Build history of the part. All positions in model axes, mm. Coordinates: 2 decimals unless noted, no trailing zeros. Loops run counter-clockwise (first coordinate to the right, second up) from the corner with the lowest first, then second, coordinate; pieces in that order, holes last.
(1) Slice it at D-D (z = 1.4). Give the cut face in (x, y), and give its area (3 significant figures).
(2) Slice it at C-C (y = -0.25). Give the cut face in (x, z), and give its area (3 significant figures).
(3) Wall check: L1, parallel to X at y = -0.1, z = 0; L2, parallel to Z at x = 14, y = 0.2; L3, parallel to X at y = 0.4, z = -1.05. Give the ranges that are in metal, low to high.
(4) Slice it at A-A (z = 0). Give the cut face in (x, y), and give its area (3 significant figures).
(5) Slice it at B-B (x = 0). Give the cut face in (y, z), and give its area (3 significant figures).
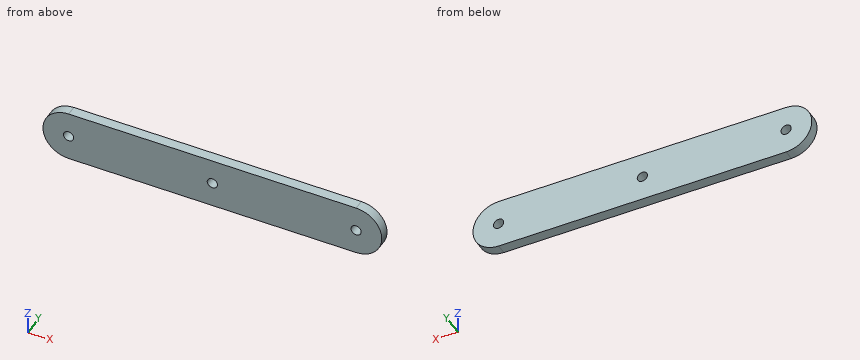
from build123d import *

# Parameters (mm, degrees)
SCHIZZO1_R                   = 0.5
ESTRUSIONE_ESTRUSIONE3_DEPTH = 0.5


with BuildPart() as part:
    # Schizzo1 → Estrusione-Estrusione3 (new body, symmetric)
    with BuildSketch(Plane(origin=(0, 0, 0), x_dir=(1, 0, 0), z_dir=(0, 1, 0))):
        with BuildLine():
            Line((-14, 2.5), (14, 2.5))
            ThreePointArc((14, 2.5), (16.5, 0), (14, -2.5))
            Line((14, -2.5), (-14, -2.5))
            ThreePointArc((-14, -2.5), (-16.5, 0), (-14, 2.5))
        make_face()
        Circle(SCHIZZO1_R, mode=Mode.SUBTRACT)
        with Locations((-14, 0)):
            Circle(SCHIZZO1_R, mode=Mode.SUBTRACT)
        with Locations((14, 0)):
            Circle(SCHIZZO1_R, mode=Mode.SUBTRACT)
    extrude(amount=ESTRUSIONE_ESTRUSIONE3_DEPTH, both=True)


solid = part.part
Response values:
1. outline: (-16.07, -0.5) - (16.07, -0.5) - (16.07, 0.5) - (-16.07, 0.5) - close
1. area: 32.1 mm2
2. outline: (-14, -2.5) - (14, -2.5) arc R2.5 ccw to (14, 2.5) - (-14, 2.5) arc R2.5 ccw to start; hole circle Ø1 at (-14, 0); hole circle Ø1 at (0, 0); hole circle Ø1 at (14, 0)
2. area: 157 mm2
3. L1: x = -16.5 to -14.5, -13.5 to -0.5, 0.5 to 13.5, 14.5 to 16.5
3. L2: z = -2.5 to -0.5, 0.5 to 2.5
3. L3: x = -16.27 to 16.27
4. outline: (-16.5, -0.5) - (-14.5, -0.5) - (-14.5, 0.5) - (-16.5, 0.5) - close; (-13.5, -0.5) - (-0.5, -0.5) - (-0.5, 0.5) - (-13.5, 0.5) - close; (0.5, -0.5) - (13.5, -0.5) - (13.5, 0.5) - (0.5, 0.5) - close; (14.5, -0.5) - (16.5, -0.5) - (16.5, 0.5) - (14.5, 0.5) - close
4. area: 30.0 mm2
5. outline: (-0.5, -2.5) - (0.5, -2.5) - (0.5, -0.5) - (-0.5, -0.5) - close; (-0.5, 0.5) - (0.5, 0.5) - (0.5, 2.5) - (-0.5, 2.5) - close
5. area: 4.00 mm2
